```python
from build123d import *

# Parameters (mm, degrees)
BOSS_EXTRUDE1_DEPTH = 18
BOSS_EXTRUDE2_DEPTH = 28
SKETCH4_R           = 3
BOSS_EXTRUDE3_DEPTH = 6


with BuildPart() as part:
    # Sketch1 → Boss-Extrude1 (new body)
    with BuildSketch(Plane.XY):
        Polygon((-40, 34), (-27.876000888, 8), (0, 8), (0, 16), (-24, 16), (-24, 34), align=None)
    extrude(amount=-BOSS_EXTRUDE1_DEPTH)

    # Sketch1_4 → Boss-Extrude2 (add)
    with BuildSketch(Plane.XY):
        Polygon((-78, 0), (0, 0), (0, 8), (-27.876000888, 8), (-40, 34), (-51.191383796, 58), (-64.786000601, 51.660726074), (-54.622678955, 29.865412469), (-59.154217891, 27.75232116), (-69.317539536, 49.547634765), (-78, 45.498936959), align=None)
    extrude(amount=-BOSS_EXTRUDE2_DEPTH)

    # Sketch4 → Boss-Extrude3 (add)
    with BuildSketch(Plane(origin=(-31.358387135, 67.248278227, 0), x_dir=(0.9063077870366475, 0.42261826174070477, 0), z_dir=(-0.42261826174070477, 0.9063077870366475, 0))):
        with Locations((-29.383290582, 7)):
            Circle(SKETCH4_R)
        with Locations((-29.383290582, 21)):
            Circle(SKETCH4_R)
    extrude(amount=BOSS_EXTRUDE3_DEPTH)


solid = part.part
```
Work out the finished part from the listing and answer in its coordinate system (mm). A direction names the side the tool comes from. Coordinates: 2 decimals unless noted, no trailing zeros. Write each loop counter-clockwise with the first axis right and the second up, starting at its lowest first coordinate (ties: lowest second). Pieces come first, ordered by that corner, then holes.
Q1. A cutting plane is placed at A-A, the plane z = -11.5. Give the vertices of the cut face in (x, y), then the cut area to 3 significant figures.
Q2. Which of the six approach directions +Z, -Z, +X, -X, +Y, -Y give full straight-line access (tool end or side, diameter ignored) to faces 1 (the face through (-48, 23, 0)), 2 (the face through (-32, 34, -9)), 3 (the face through (-64.165, 38.497, -13.804)), 4 (the face through (-25, 18, -18)), 5 (the face through (-73.6, 47.55, -13.8))?
Q3. A cutting plane is placed at C-C, the plane y = 14. Give the vertices of the cut face in (x, z), then the cut area to 3 significant figures.
Q4. Determine the mould class of faces 6 (the face through (-57, 23, -28)), 7 (the face through (-56.86, 28.82, -13.8)), 8 (the face through (-78, 23, -14)) for opening direction X: released by +X, released by -X, zero draft, split by the parting line, or undercut.
Q5. Find the intervals of material crossed by line 1 (Y direction, x = -34, z = -17.5); line 2 (X direction, y = 18, z = -6.5); line 3 (Z direction, x = -28.5, y = 10.5), in increasing order.
Q6. A cutting plane is placed at D-D, the plane z = -26. Give the vertices of the cut face in (x, y).
Q7. Each of these flat-tipped pins is pushed along its axis until it touches: pin 1 Ø8 at (x, z) = (-32.5, -5) entering from +Y; pin 2 Ø8 at (y, z) = (28.5, -3) entering from +X; pin 3 Ø11 at (x, z) = (-17.5, -21) entering from +Y. Where does it stop, or does it pass through?
Q8. A cutting plane is placed at B-B, the plane x = -8. Give the vertices of the cut face in (y, z), then the cut area to 3 significant figures.
Findings below:
1. outline: (-78, 0) - (0, 0) - (0, 16) - (-24, 16) - (-24, 34) - (-40, 34) - (-51.19, 58) - (-64.79, 51.66) - (-54.62, 29.87) - (-59.15, 27.75) - (-69.32, 49.55) - (-78, 45.5) - close
1. area: 2,710 mm2
2. face 1: +Z, +X, -X, +Y, -Y
2. face 2: +Z, -Z, +X, +Y
2. face 3: +Z, -Z
2. face 4: -Z, +X, +Y
2. face 5: +Z, -Z, -X, +Y
3. outline: (-78, -28) - (-30.67, -28) - (-30.67, -18) - (0, -18) - (0, 0) - (-78, 0) - close
3. area: 1,880 mm2
4. face 6: zero draft
4. face 7: undercut
4. face 8: released by -X
5. line 1: y = 0 to 34
5. line 2: x = -78 to -24
5. line 3: z = -18 to 0
6. outline: (-78, 0) - (0, 0) - (0, 8) - (-27.88, 8) - (-51.19, 58) - (-64.79, 51.66) - (-54.62, 29.87) - (-59.15, 27.75) - (-69.32, 49.55) - (-78, 45.5) - close
7. pin 1: stops at y = 34
7. pin 2: stops at x = -24
7. pin 3: stops at y = 16
8. outline: (0, -28) - (8, -28) - (8, -18) - (16, -18) - (16, 0) - (0, 0) - close
8. area: 368 mm2
